Geometry: final body of the model. Coordinates: model frame, mm. A direction names the side the tool comes from. Coordinates: 2 decimals unless noted, no trailing zeros. Order: outer loops, then holes, each group sorted by start corner. A loop starts at its lowest first (then second) coordinate and runs counter-clockwise, first axis right, second up. Notation, with made-up numbers: M 34,52 L 71,52 A25 cw 71,70 Z; hole C 47.5,89 d11. An arc over 180 degrees is marked long. Write item = value, one per line.
from build123d import *

# Parameters (mm, degrees)
F0_W         = 50
F0_H         = 55
F0_R         = 15
F0_R_2       = 12.5
F1_DEPTH     = 25
F2_DEPTH     = 50
F3_T1_DEPTH  = 40
F3_T3_DEPTH  = 45
F3_T5_DEPTH  = 15
F3_S9_W      = 5.1
F3_S9_H      = 5.1
F3_T10_DEPTH = 5.1
F3_S15_W     = 5.1
F3_S15_H     = 5.1
F3_T16_DEPTH = 5.1
F3_S21_W     = 5.1
F3_S21_H     = 5.1
F3_T22_DEPTH = 5.1
F3_S27_W     = 5.1
F3_S27_H     = 5.1
F3_T28_DEPTH = 5.1
F3_S33_W     = 5.1
F3_S33_H     = 5.1
F3_T34_DEPTH = 5.1
F3_S39_W     = 5.1
F3_S39_H     = 5.1
F3_T40_DEPTH = 5.1
F3_S45_W     = 5.1
F3_S45_H     = 5.1
F3_T46_DEPTH = 5.1
F3_S51_W     = 5.1
F3_S51_H     = 5.1
F3_T52_DEPTH = 5.1


# Not quite as in the source:
# - a fillet or chamfer that OpenCascade refuses, or shapes differently, is made with other operations: its cross-section is extruded or revolved along the edge and cut away or added


with BuildPart() as f1:
    # F0 (on Top) → F1 (new body)
    with BuildSketch(Plane.XY):
        with Locations((-25, 27.5)):
            Rectangle(F0_W, F0_H)
        with Locations((-25, 27.5)):
            Circle(F0_R, mode=Mode.SUBTRACT)
        with Locations((-25, 27.5)):
            Circle(F0_R)
        with Locations((-25, 27.5)):
            Circle(F0_R_2, mode=Mode.SUBTRACT)
        with Locations((-25, 27.5)):
            Circle(F0_R_2)
    extrude(amount=F1_DEPTH)

    # F0 (on Top) → F2 (join)
    with BuildSketch(Plane.XY):
        with Locations((-25, 27.5)):
            Circle(F0_R)
        with Locations((-25, 27.5)):
            Circle(F0_R_2, mode=Mode.SUBTRACT)
    extrude(amount=F2_DEPTH)

    # F3: fillet of radius 5 on 13 edges, made by hand

    # F3_s2 → F3_t1 (cut)
    with BuildSketch(Plane.YZ.offset(-45)):
        with BuildLine():
            ThreePointArc((55, 20), (53.5355339059, 23.5355339059), (50, 25))
            Line((50, 25), (55, 25))
            Line((55, 25), (55, 20))
        make_face()
        with BuildLine():
            ThreePointArc((5, 0), (1.4644660941, 1.4644660941), (0, 5))
            Line((0, 5), (0, 0))
            Line((0, 0), (5, 0))
        make_face()
        with BuildLine():
            ThreePointArc((5, 25), (1.4644660941, 23.5355339059), (0, 20))
            Line((0, 20), (0, 25))
            Line((0, 25), (5, 25))
        make_face()
        with BuildLine():
            ThreePointArc((55, 5), (53.5355339059, 1.4644660941), (50, 0))
            Line((50, 0), (55, 0))
            Line((55, 0), (55, 5))
        make_face()
    extrude(amount=F3_T1_DEPTH, mode=Mode.SUBTRACT)

    # F3_s4 → F3_t3 (cut)
    with BuildSketch(Plane.XZ.offset(-50)):
        with BuildLine():
            ThreePointArc((-50, 20), (-48.5355339059, 23.5355339059), (-45, 25))
            Line((-45, 25), (-50, 25))
            Line((-50, 25), (-50, 20))
        make_face()
        with BuildLine():
            ThreePointArc((0, 5), (-1.4644660941, 1.4644660941), (-5, 0))
            Line((-5, 0), (0, 0))
            Line((0, 0), (0, 5))
        make_face()
        with BuildLine():
            ThreePointArc((0, 20), (-1.4644660941, 23.5355339059), (-5, 25))
            Line((-5, 25), (0, 25))
            Line((0, 25), (0, 20))
        make_face()
        with BuildLine():
            ThreePointArc((-50, 5), (-48.5355339059, 1.4644660941), (-45, 0))
            Line((-45, 0), (-50, 0))
            Line((-50, 0), (-50, 5))
        make_face()
    extrude(amount=F3_T3_DEPTH, mode=Mode.SUBTRACT)

    # F3_s6 → F3_t5 (cut)
    with BuildSketch(Plane.XY.offset(5)):
        with BuildLine():
            ThreePointArc((-50, 5), (-48.5355339059, 1.4644660941), (-45, 0))
            Line((-45, 0), (-50, 0))
            Line((-50, 0), (-50, 5))
        make_face()
        with BuildLine():
            ThreePointArc((0, 5), (-1.4644660941, 1.4644660941), (-5, 0))
            Line((-5, 0), (0, 0))
            Line((0, 0), (0, 5))
        make_face()
        with BuildLine():
            ThreePointArc((-5, 55), (-1.4644660941, 53.5355339059), (0, 50))
            Line((0, 50), (0, 55))
            Line((0, 55), (-5, 55))
        make_face()
        with BuildLine():
            ThreePointArc((-45, 55), (-48.5355339059, 53.5355339059), (-50, 50))
            Line((-50, 50), (-50, 55))
            Line((-50, 55), (-45, 55))
        make_face()
    extrude(amount=F3_T5_DEPTH, mode=Mode.SUBTRACT)


with BuildPart() as f3_tool8:
    # F3_s9 → F3_t10 (new body)
    with BuildSketch(Plane.XZ.offset(-50)):
        with Locations((-2.45, 22.55)):
            Rectangle(F3_S9_W, F3_S9_H)
    extrude(amount=-F3_T10_DEPTH)

    # F3_s11 → F3_t12 (revolve, cut)
    with BuildSketch(Plane(origin=(-5, 50, 20), x_dir=(-0.7071067812, 0, -0.7071067812), z_dir=(0.7071067812, 0, -0.7071067812))):
        with BuildLine():
            ThreePointArc((0, -5), (5, 0), (0, 5))
            Line((0, 5), (0, -5))
        make_face()
    revolve(axis=Axis((-5, 50, 20), (0, 1, 0)), mode=Mode.SUBTRACT)


with BuildPart() as f1_1:
    add(f1.part)

    # F3_t7: cut F3_tool8
    add(f3_tool8.part, mode=Mode.SUBTRACT)


with BuildPart() as f3_tool14:
    # F3_s15 → F3_t16 (new body)
    with BuildSketch(Plane.XZ.offset(-50)):
        with Locations((-47.55, 22.55)):
            Rectangle(F3_S15_W, F3_S15_H)
    extrude(amount=-F3_T16_DEPTH)

    # F3_s17 → F3_t18 (revolve, cut)
    with BuildSketch(Plane(origin=(-45, 50, 20), x_dir=(0.7071067812, 0, -0.7071067812), z_dir=(0.7071067812, 0, 0.7071067812))):
        with BuildLine():
            ThreePointArc((0, -5), (5, 0), (0, 5))
            Line((0, 5), (0, -5))
        make_face()
    revolve(axis=Axis((-45, 50, 20), (0, 1, 0)), mode=Mode.SUBTRACT)


with BuildPart() as f1_2:
    add(f1_1.part)

    # F3_t13: cut F3_tool14
    add(f3_tool14.part, mode=Mode.SUBTRACT)


with BuildPart() as f3_tool20:
    # F3_s21 → F3_t22 (new body)
    with BuildSketch(Plane.YZ.offset(-45)):
        with Locations((2.45, 22.55)):
            Rectangle(F3_S21_W, F3_S21_H)
    extrude(amount=-F3_T22_DEPTH)

    # F3_s23 → F3_t24 (revolve, cut)
    with BuildSketch(Plane(origin=(-45, 5, 20), x_dir=(0, 0.7071067812, -0.7071067812), z_dir=(0, 0.7071067812, 0.7071067812))):
        with BuildLine():
            ThreePointArc((0, -5), (5, 0), (0, 5))
            Line((0, 5), (0, -5))
        make_face()
    revolve(axis=Axis((-45, 5, 20), (-1, 0, 0)), mode=Mode.SUBTRACT)


with BuildPart() as f1_3:
    add(f1_2.part)

    # F3_t19: cut F3_tool20
    add(f3_tool20.part, mode=Mode.SUBTRACT)


with BuildPart() as f3_tool26:
    # F3_s27 → F3_t28 (new body)
    with BuildSketch(Plane.YZ.offset(-45)):
        with Locations((2.45, 2.45)):
            Rectangle(F3_S27_W, F3_S27_H)
    extrude(amount=-F3_T28_DEPTH)

    # F3_s29 → F3_t30 (revolve, cut)
    with BuildSketch(Plane(origin=(-45, 5, 5), x_dir=(0, 0.7071067812, 0.7071067812), z_dir=(0, -0.7071067812, 0.7071067812))):
        with BuildLine():
            ThreePointArc((0, -5), (5, 0), (0, 5))
            Line((0, 5), (0, -5))
        make_face()
    revolve(axis=Axis((-45, 5, 5), (-1, 0, 0)), mode=Mode.SUBTRACT)


with BuildPart() as f1_4:
    add(f1_3.part)

    # F3_t25: cut F3_tool26
    add(f3_tool26.part, mode=Mode.SUBTRACT)


with BuildPart() as f3_tool32:
    # F3_s33 → F3_t34 (new body)
    with BuildSketch(Plane.YZ.offset(-5)):
        with Locations((2.45, 2.45)):
            Rectangle(F3_S33_W, F3_S33_H)
    extrude(amount=F3_T34_DEPTH)

    # F3_s35 → F3_t36 (revolve, cut)
    with BuildSketch(Plane(origin=(-5, 5, 5), x_dir=(0, 0.7071067812, 0.7071067812), z_dir=(0, 0.7071067812, -0.7071067812))):
        with BuildLine():
            ThreePointArc((0, -5), (5, 0), (0, 5))
            Line((0, 5), (0, -5))
        make_face()
    revolve(axis=Axis((-5, 5, 5), (1, 0, 0)), mode=Mode.SUBTRACT)


with BuildPart() as f1_5:
    add(f1_4.part)

    # F3_t31: cut F3_tool32
    add(f3_tool32.part, mode=Mode.SUBTRACT)


with BuildPart() as f3_tool38:
    # F3_s39 → F3_t40 (new body)
    with BuildSketch(Plane.YZ.offset(-5)):
        with Locations((2.45, 22.55)):
            Rectangle(F3_S39_W, F3_S39_H)
    extrude(amount=F3_T40_DEPTH)

    # F3_s41 → F3_t42 (revolve, cut)
    with BuildSketch(Plane(origin=(-5, 5, 20), x_dir=(0, 0.7071067812, -0.7071067812), z_dir=(0, -0.7071067812, -0.7071067812))):
        with BuildLine():
            ThreePointArc((0, -5), (5, 0), (0, 5))
            Line((0, 5), (0, -5))
        make_face()
    revolve(axis=Axis((-5, 5, 20), (1, 0, 0)), mode=Mode.SUBTRACT)


with BuildPart() as f1_6:
    add(f1_5.part)

    # F3_t37: cut F3_tool38
    add(f3_tool38.part, mode=Mode.SUBTRACT)


with BuildPart() as f3_tool44:
    # F3_s45 → F3_t46 (new body)
    with BuildSketch(Plane.XZ.offset(-50)):
        with Locations((-2.45, 2.45)):
            Rectangle(F3_S45_W, F3_S45_H)
    extrude(amount=-F3_T46_DEPTH)

    # F3_s47 → F3_t48 (revolve, cut)
    with BuildSketch(Plane(origin=(-5, 50, 5), x_dir=(-0.7071067812, 0, 0.7071067812), z_dir=(-0.7071067812, 0, -0.7071067812))):
        with BuildLine():
            ThreePointArc((0, -5), (5, 0), (0, 5))
            Line((0, 5), (0, -5))
        make_face()
    revolve(axis=Axis((-5, 50, 5), (0, 1, 0)), mode=Mode.SUBTRACT)


with BuildPart() as f1_7:
    add(f1_6.part)

    # F3_t43: cut F3_tool44
    add(f3_tool44.part, mode=Mode.SUBTRACT)


with BuildPart() as f3_tool50:
    # F3_s51 → F3_t52 (new body)
    with BuildSketch(Plane.XZ.offset(-50)):
        with Locations((-47.55, 2.45)):
            Rectangle(F3_S51_W, F3_S51_H)
    extrude(amount=-F3_T52_DEPTH)

    # F3_s53 → F3_t54 (revolve, cut)
    with BuildSketch(Plane(origin=(-45, 50, 5), x_dir=(0.7071067812, 0, 0.7071067812), z_dir=(-0.7071067812, 0, 0.7071067812))):
        with BuildLine():
            ThreePointArc((0, -5), (5, 0), (0, 5))
            Line((0, 5), (0, -5))
        make_face()
    revolve(axis=Axis((-45, 50, 5), (0, 1, 0)), mode=Mode.SUBTRACT)


with BuildPart() as f1_8:
    add(f1_7.part)

    # F3_t49: cut F3_tool50
    add(f3_tool50.part, mode=Mode.SUBTRACT)

    # F3_s55 → F3_t56 (revolve, cut)
    with BuildSketch(Plane.XZ.offset(-27.5)):
        with BuildLine():
            ThreePointArc((-10, 50), (-11.8301270189, 48.1698729811), (-12.5, 45.6698729811))
            Line((-12.5, 45.6698729811), (-12.5, 50))
            Line((-12.5, 50), (-10, 50))
        make_face()
    revolve(axis=Axis((-25, 27.5, 50), (0, 0, 1)), mode=Mode.SUBTRACT)


solid = f1_8.part
1) Section D-D, the plane x = -43.5. Return loops of the section in (y, z), and give its area (3 significant figures).
Numbers:
outline = M 0,5 A5 ccw 5,0 L 50,0 A5 ccw 55,5 L 55,20 A5 ccw 50,25 L 5,25 A5 ccw 0,20 Z
area = 1,350 mm²
2) Section B-B, the plane y = 27.5. Return loops of the section in (x, z), and give its area (3 significant figures).
Numbers:
outline = M -50,5 A5 ccw -45,0 L -5,0 A5 ccw 0,5 L 0,20 A5 ccw -5,25 L -10,25 L -10,50 A5 ccw -12.5,45.67 L -12.5,25 L -37.5,25 L -37.5,45.67 A5 ccw -40,50 L -40,25 L -45,25 A5 ccw -50,20 Z
area = 1,350 mm²
3) Line query: L1, parallel to X at y = 28, z = 32.5; L2, parallel to Y at x = -25, z = 39; L3, parallel to Z at x = -35, y = 42. Output: solid intervals per line, ascending.
Numbers:
L1 = -39.99 to -37.49, -12.51 to -10.01
L2 = 12.5 to 15, 40 to 42.5
L3 = 0 to 25
4) Set-up query: faces 1 (the face through (-25, 28, 0)), 2 (the face through (-25, 43, 25)). Return all of +Z, -Z, +X, -X, +Y, -Y with unobstructed straight access to the full face (end or side cutting, diameter ignored); none if empty.
Numbers:
face_1 = -Z, +X, -X, +Y, -Y
face_2 = +Z
5) Section C-C, the plane z = 32. Return loops of the section in (x, y), and give its area (3 significant figures).
Numbers:
outline = C -25,27.5 d30; hole C -25,27.5 d25
area = 216 mm²
6) Section A-A, the plane x = -25. Return loops of the section in (y, z), and give its area (3 significant figures).
Numbers:
outline = M 0,5 A5 ccw 5,0 L 50,0 A5 ccw 55,5 L 55,20 A5 ccw 50,25 L 42.5,25 L 42.5,50 A5 ccw 40,45.67 L 40,25 L 15,25 L 15,45.67 A5 ccw 12.5,50 L 12.5,25 L 5,25 A5 ccw 0,20 Z
area = 1,470 mm²
7) Pin query (flat end, axial travel): pin 1 (2 mm diameter, centred on y = 33, z = 42, fed in from -X); pin 2 (1.5 mm diameter, centred on x = -12, z = 37, fed in from -Y); pin 3 (2 mm diameter, centred on x = -43.5, y = 23, fed in from +Z). Return the tip coordinate at first contact, or that it passes through.
Numbers:
pin_1 = -39.31
pin_2 = 18.84
pin_3 = 25
8) Mould query, pull axis X, two halves, no side actions, for faces 3 (the face through (-25, 28, 25)), 4 (the face through (-35, 20, 35)), 5 (the face through (-1, 28, 2)), 6 (the face through (-25, 2, 1)). Classes: pulls with the +X half, pulls with the -X half, needs draft (parallel to the pull), parting line crosses it, or undercut.
Numbers:
face_3 = undercut
face_4 = undercut
face_5 = pulls with the +X half
face_6 = needs draft
